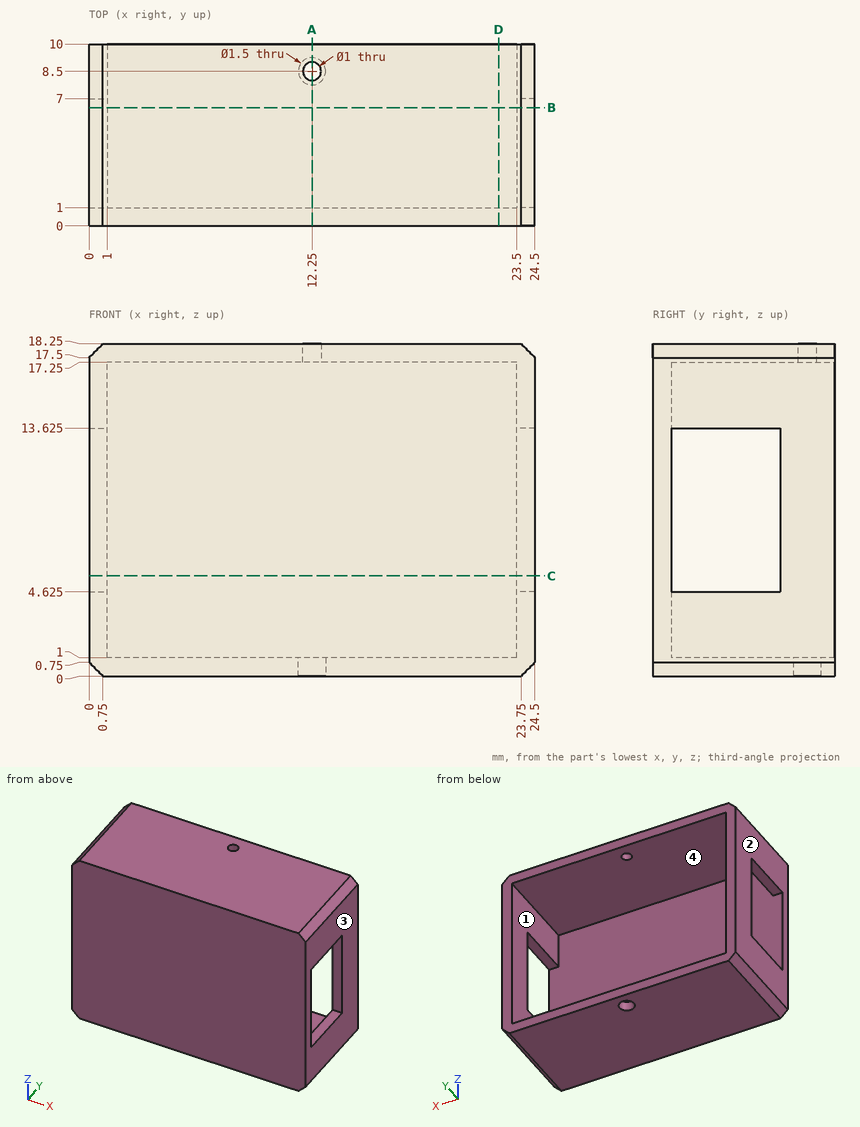
Source: three-view drawing plus pictorial views. Frame: mm from the lowest corner of the part. Coordinates: 2 decimals unless noted, no trailing zeros. Write each loop counter-clockwise with the first axis right and the second up, starting at its lowest first coordinate (ties: lowest second). Pieces come first, ordered by that corner, then holes. Notation, with made-up numbers: (-16, 67) -> (-2, 67) arc R30 cw to (-2, 89) -> close; hole circle Ø2 at (9.25, 47.25). An arc over 180 degrees is marked (long way). Answer as a JSON object with one key per item and string values.
1. Section B-B on y = 6.5. Return the cut outline in (x, z) (3 decimals).
Result set:
{"outline": "(0, 0.75) -> (0.75, 0) -> (23.75, 0) -> (24.5, 0.75) -> (24.5, 4.625) -> (23.5, 4.625) -> (23.5, 1) -> (1, 1) -> (1, 4.625) -> (0, 4.625) -> close; (0, 13.625) -> (1, 13.625) -> (1, 17.25) -> (23.5, 17.25) -> (23.5, 13.625) -> (24.5, 13.625) -> (24.5, 17.5) -> (23.75, 18.25) -> (0.75, 18.25) -> (0, 17.5) -> close"}
2. Section D-D on x = 22.5. Return the cut outline in (y, z).
Result set:
{"outline": "(0, 0) -> (10, 0) -> (10, 1) -> (1, 1) -> (1, 17.25) -> (10, 17.25) -> (10, 18.25) -> (0, 18.25) -> close"}
3. Material intervals for line 1 (Z direction, x = 7, y = 5.5); line 2 (X direction, y = 3, z = 13.75); line 3 (Y direction, x = 12.25, z = 17.75), sorted ascending. Write a range as from..to.
Result set:
{"line 1": "z = 0..1, 17.25..18.25", "line 2": "x = 0..1, 23.5..24.5", "line 3": "y = 0..8, 9..10"}
4. First-contact query: P1, Ø5, axis at x = 16.5, z = 14.5, coming from the +Y side. Flat tip, straight axial feed; report the tip coordinate or a pass-through.
Result set:
{"P1": "stops at y = 1"}
5. Mould query, pull axis X, two halves, no side actions, for the marked faces 1, 2, 3 and 4. Classes: released by +X, released by -X, zero draft, split by the parting line, or undercut.
Result set:
{"face 1": "undercut", "face 2": "released by -X", "face 3": "released by +X", "face 4": "undercut"}
6. Section C-C on z = 5.5. Return the cut outline in (x, y).
Result set:
{"outline": "(0, 0) -> (24.5, 0) -> (24.5, 1) -> (0, 1) -> close; (0, 7) -> (1, 7) -> (1, 10) -> (0, 10) -> close; (23.5, 7) -> (24.5, 7) -> (24.5, 10) -> (23.5, 10) -> close"}
7. Section A-A on x = 12.25. Return the cut outline in (y, z), then the cut area to 4 significant figures.
Result set:
{"outline": "(0, 0) -> (7.75, 0) -> (7.75, 1) -> (1, 1) -> (1, 17.25) -> (8, 17.25) -> (8, 18.25) -> (0, 18.25) -> close; (9, 17.25) -> (10, 17.25) -> (10, 18.25) -> (9, 18.25) -> close; (9.25, 0) -> (10, 0) -> (10, 1) -> (9.25, 1) -> close", "area": "33.75 mm2"}
